from build123d import *

# Parameters (mm, degrees)
SKETCH1_W                 = 45
SKETCH1_H                 = 45
BASEPLATE_DEPTH           = 2
SKETCH2_R                 = 0.25
PINFIN_DEPTH              = 2
PINFIN_PATTERN_COUNT      = 5
PINFIN_PATTERN_PITCH      = 1
PINFIN_PATTERN_COUNT_DIR2 = 5
PINFIN_PATTERN_PITCH_DIR2 = 1


with BuildPart() as part:
    # Sketch1 → Baseplate (new body)
    with BuildSketch(Plane(origin=(0, 0, 0), x_dir=(1, 0, 0), z_dir=(0, 1, 0))):
        Rectangle(SKETCH1_W, SKETCH1_H)
    extrude(amount=BASEPLATE_DEPTH)

    # Sketch2 → Pinfin (add)
    with BuildSketch(Plane(origin=(0, 2, 0), x_dir=(1, 0, 0), z_dir=(0, 1, 0))):
        with Locations(Location((-2, -2, 0), (0, 0, 270))):
            Circle(SKETCH2_R)
    pinfin = extrude(amount=PINFIN_DEPTH)

    # Pinfin Pattern: Pinfin 5 × 5
    with Locations(*[(j * PINFIN_PATTERN_PITCH_DIR2, 0, -i * PINFIN_PATTERN_PITCH) for i in range(PINFIN_PATTERN_COUNT) for j in range(PINFIN_PATTERN_COUNT_DIR2) if (i, j) != (0, 0)]):
        add(pinfin)


solid = part.part
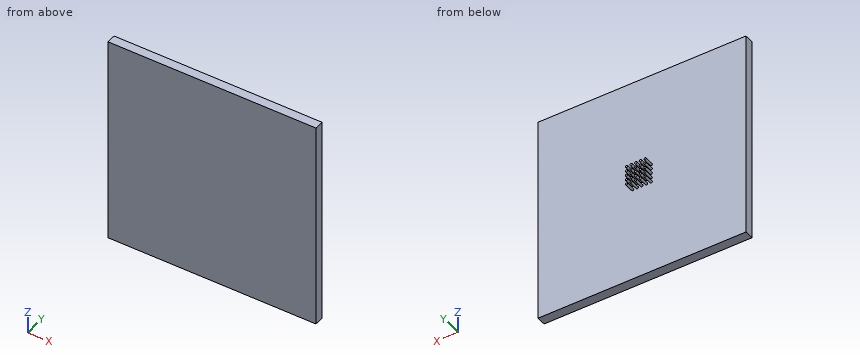
CAD build for the part. Positions are in the model's coordinates, mm. Give positions to 0.01 mm unless a question says otherwise; leave off trailing zeros. Loops run counter-clockwise (first coordinate to the right, second up) from the corner with the lowest first, then second, coordinate; pieces in that order, holes last. Notation, with made-up numbers: M 74,65 L 129,65 A30 ccw 129,92 Z; hole C 62.5,24.5 d3. An arc over 180 degrees is marked long. Write each question's results on one line, items separated by ' | '.
Q1. Flat gauge pin, fed straight in: P1, Ø1.5, axis at x = 5, z = 16.5, coming from the +Y side. Where does the tip first touch, or does it go through?
Geometry check:
P1: stops at y = 2
Q2. Band-saw the part on A-A on y = 3.4. Give the number of separate pieces and of enclosed holes in the cut face, and give its area (3 significant figures).
Geometry check:
separate pieces: 25 | enclosed holes: 0 | area: 4.91 mm²
Q3. Probe probe 1 along Y at (x, z) = (14.5, 14.5). List the from-to ranges inside material, lowest first.
Geometry check:
probe 1: y = 0 to 2
Q4. Band-saw the part on C-C on x = -10.5. Write the cut outline in (y, z), and give its area (3 significant figures).
Geometry check:
outline: M 0,-22.5 L 2,-22.5 L 2,22.5 L 0,22.5 Z | area: 90.0 mm²
Q5. Band-saw the part on B-B on z = 19.5. Write the cut outline in (x, y).
Geometry check:
outline: M -22.5,0 L 22.5,0 L 22.5,2 L -22.5,2 Z
